```python
from build123d import *

# Parameters (mm, degrees)
SKETCH3_R           = 1.4224
BOSS_EXTRUDE1_DEPTH = 1.190625
FILLET1_R           = 0.79375
CHAMFER1_SIZE       = 0.127


with BuildPart() as part:
    # Sketch3 → Boss-Extrude1 (new body, symmetric)
    with BuildSketch(Plane(origin=(0, 0, 0), x_dir=(1, 0, 0), z_dir=(0, 1, 0))):
        Polygon((1.833087105, 3.175), (-1.833087105, 3.175), (-3.666174209, 0), (-1.833087105, -3.175), (1.833087105, -3.175), (3.666174209, 0), align=None)
        Circle(SKETCH3_R, mode=Mode.SUBTRACT)
    extrude(amount=BOSS_EXTRUDE1_DEPTH, both=True)

    # Fillet1
    fillet1_edges = [part.edges().sort_by_distance(p)[0] for p in [
        (3.666174209, 0, 0),
        (1.833087105, 0, 3.175),
        (-1.833087105, 0, 3.175),
        (-3.666174209, 0, 0),
        (-1.833087105, 0, -3.175),
        (1.833087105, 0, -3.175),
    ]]
    fillet(fillet1_edges, radius=FILLET1_R)

    # Chamfer1
    chamfer1_edges = [part.edges().sort_by_distance(p)[0] for p in [
        (-1.4224, -1.190625, 0),
        (-1.4224, 1.190625, 0),
        (2.749630657, -1.190625, -1.5875),
        (2.749630657, 1.190625, -1.5875),
        (2.749630657, -1.190625, 1.5875),
        (0, -1.190625, 3.175),
        (-2.749630657, -1.190625, 1.5875),
        (-2.749630657, -1.190625, -1.5875),
        (0, -1.190625, -3.175),
        (-1.771690329, -1.190625, 3.068657664),
        (1.771690329, -1.190625, -3.068657664),
        (-1.771690329, -1.190625, -3.068657664),
        (-3.543380657, -1.190625, 0),
        (1.771690329, -1.190625, 3.068657664),
        (3.543380657, -1.190625, 0),
        (2.749630657, 1.190625, 1.5875),
        (0, 1.190625, -3.175),
        (-2.749630657, 1.190625, -1.5875),
        (-2.749630657, 1.190625, 1.5875),
        (0, 1.190625, 3.175),
        (-1.771690329, 1.190625, 3.068657664),
        (1.771690329, 1.190625, -3.068657664),
        (-1.771690329, 1.190625, -3.068657664),
        (-3.543380657, 1.190625, 0),
        (1.771690329, 1.190625, 3.068657664),
        (3.543380657, 1.190625, 0),
    ]]
    chamfer(chamfer1_edges, length=CHAMFER1_SIZE)


solid = part.part
```
Source: CAD feature listing. Evaluate the final solid. Frame: model axes, mm. Give positions to 0.01 mm unless a question says otherwise; leave off trailing zeros. Loops run counter-clockwise (first coordinate to the right, second up) from the corner with the lowest first, then second, coordinate; pieces in that order, holes last. Notation, with made-up numbers: (44, 19) - (89, 19) arc R33 cw to (89, 58) - close; hole circle Ø8 at (23.5, 55). An arc over 180 degrees is marked (long way). Use CSV: the item, a comma, the result in double quotes. Start each with the question number.
1. Pin query (flat end, axial travel): pin 1 (2.5 mm diameter, centred on x = 0, z = 0, fed in from +Y). Return the tip coordinate at first contact, or that it passes through.
2. Draft query along Z for faces 1 (the flat face through (-2, 1.191, 0)), 2 (the flat face through (0, 0, 3.175)), 3 (the cylindrical face through (-0.31, -0.01, 1.39)). Return one class per face: +Z half, -Z half, draft (parallel to the pull), parting line (faces both ways), or undercut.
3. Ray query, L1, parallel to X at y = 0, z = 0; L2, parallel to Z at x = 0, y = -0.4 (3 decimals); L3, parallel to Z at x = 1, y = 0.75 (3 decimals). Return the intervals inside material, ascending.
4. Section C-C (y = 0.5). Output: boundary loops of the cut face in (x, z) (1 decimal).
5. Section D-D (z = 2.5). Output: boundary loops of the cut face in (x, y).
6. Section A-A (z = 0). Output: boundary loops of the cut face in (x, y).
7. Section B-B (x = 0). Output: boundary loops of the cut face in (y, z) (3 decimals), then the cut area to 3 significant figures.
Response:
1,pin 1,"through"
2,face 1,"draft"
2,face 2,"+Z half"
2,face 3,"undercut"
3,L1,"-3.54 to -1.42, 1.42 to 3.54"
3,L2,"-3.175 to -1.422, 1.422 to 3.175"
3,L3,"-3.175 to -1.012, 1.012 to 3.175"
4,outline,"(-3.4, -0.4) - (-2.1, -2.8) arc R0.8 ccw to (-1.4, -3.2) - (1.4, -3.2) arc R0.8 ccw to (2.1, -2.8) - (3.4, -0.4) arc R0.8 ccw to (3.4, 0.4) - (2.1, 2.8) arc R0.8 ccw to (1.4, 3.2) - (-1.4, 3.2) arc R0.8 ccw to (-2.1, 2.8) - (-3.4, 0.4) arc R0.8 ccw to start; hole circle Ø2.8 at (0, 0)"
5,outline,"(-2.22, -1.06) - (-2.08, -1.19) - (2.08, -1.19) - (2.22, -1.06) - (2.22, 1.06) - (2.08, 1.19) - (-2.08, 1.19) - (-2.22, 1.06) - close"
6,outline,"(-3.54, -1.06) - (-3.42, -1.19) - (-1.55, -1.19) - (-1.42, -1.06) - (-1.42, 1.06) - (-1.55, 1.19) - (-3.42, 1.19) - (-3.54, 1.06) - close; (1.42, -1.06) - (1.55, -1.19) - (3.42, -1.19) - (3.54, -1.06) - (3.54, 1.06) - (3.42, 1.19) - (1.55, 1.19) - (1.42, 1.06) - close"
7,outline,"(-1.191, -3.048) - (-1.064, -3.175) - (1.064, -3.175) - (1.191, -3.048) - (1.191, -1.549) - (1.064, -1.422) - (-1.064, -1.422) - (-1.191, -1.549) - close; (-1.191, 1.549) - (-1.064, 1.422) - (1.064, 1.422) - (1.191, 1.549) - (1.191, 3.048) - (1.064, 3.175) - (-1.064, 3.175) - (-1.191, 3.048) - close"
7,area,"8.28 mm²"
